Source: CAD feature listing. Evaluate the final solid. Frame: model axes, mm. Face numbers are marked on the shaded views. A direction names the side the tool comes from. Give positions to 0.01 mm unless a question says otherwise; leave off trailing zeros. Write each loop counter-clockwise with the first axis right and the second up, starting at its lowest first coordinate (ties: lowest second). Pieces come first, ordered by that corner, then holes. Notation, with made-up numbers: M 53.25,46.25 L 70.25,46.25 A26 ccw 70.25,85.25 Z; hole C 23,47.5 d4. An arc over 180 degrees is marked long. Return JSON: item names as keys, results as strings.
```python
from build123d import *

# Parameters (mm, degrees)
F2_R     = 12.5
F3_DEPTH = 12.5
F4_R     = 0.5


# Not quite as in the source:
# - the program builds the solid bodies; features that only make, move or delete a surface that nothing else refers to are left out


with BuildPart() as f1:
    # F0 (on Front) → F1 (revolve)
    with BuildSketch(Plane.XZ):
        Polygon((-14, 0), (21, 0), (21, 1.25), (19.85, 2.4), (7.3, 2.4), (6.8, 2.4), (6.4535898385, 3), (4, 3), (4, 4.8), (3.2, 5.6), (-3.2, 5.6), (-4, 4.8), (-4, 3), (-6.4535898385, 3), (-6.8, 2.4), (-7.3, 2.4), (-12.85, 2.4), (-14, 1.25), align=None)
        Polygon((7.3, 2.4), (19.85, 2.4), (19.25, 3), (7.9, 3), align=None)
        Polygon((-12.25, 3), (-12.85, 2.4), (-7.3, 2.4), (-7.9, 3), align=None)
    revolve(axis=Axis((0, 0, 0), (1, 0, 0)))

    # F2 (on Right) → F3 (cut, symmetric)
    with BuildSketch(Plane.YZ):
        Circle(F2_R)
        Polygon((5, -2.8867513459), (0, -5.7735026919), (-5, -2.8867513459), (-5, 2.8867513459), (0, 5.7735026919), (5, 2.8867513459), align=None, mode=Mode.SUBTRACT)
    extrude(amount=F3_DEPTH, both=True, mode=Mode.SUBTRACT)

    # F4
    f4_edges = [f1.edges().sort_by_distance(p)[0] for p in [
        (-4, 0, -3),
        (4, 0, -3),
    ]]
    fillet(f4_edges, radius=F4_R)


solid = f1.part
```
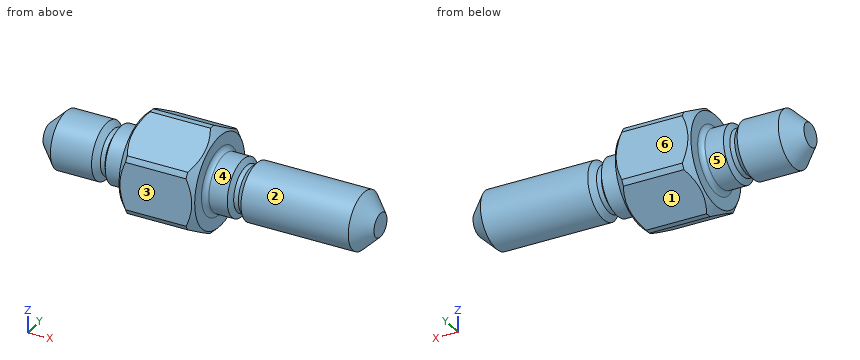
1) Cut plane A-A, the plane x = 0.5. Return the cut outline in (y, z).
Numbers:
{"outline": "M -5,-2.52 A5.6 ccw -4.68,-3.07 L -0.32,-5.59 A5.6 ccw 0.32,-5.59 L 4.68,-3.07 A5.6 ccw 5,-2.52 L 5,2.52 A5.6 ccw 4.68,3.07 L 0.32,5.59 A5.6 ccw -0.32,5.59 L -4.68,3.07 A5.6 ccw -5,2.52 Z"}
2) Set-up query: the marked faces 4, 5 and 6. Return all of +Z, -Z, +X, -X, +Y, -Y with unobstructed straight access to the full face (end or side cutting, diameter ignored); none if empty.
Numbers:
{"face 4": "+X", "face 5": "-X", "face 6": "+Z, -Z, +X, -X, +Y"}
3) Contact query for flat-ended pins moving along their axis: pin 1 Ø1.5 at (x, y) = (-4, 3.5) entering from +Z; pin 2 Ø1 at (x, z) = (-6, 1.5) entering from +Y; pin 3 Ø3 at (x, y) = (4, -2) entering from +Z. Output: stop coordinate, or through.
Numbers:
{"pin 1": "stops at z = 4.17", "pin 2": "stops at y = 2.83", "pin 3": "stops at z = 5.4"}
4) Cut plane B-B, the plane x = 13. Return the cut outline in (y, z).
Numbers:
{"outline": "C 0,0 d6"}
5) Draft query along Y for the marked faces 1, 2 and 3. Return one class per face: released by +Y, released by -Y, zero draft, split by the parting line, or undercut.
Numbers:
{"face 1": "released by +Y", "face 2": "split by the parting line", "face 3": "released by -Y"}
6) Line query: line 1 (X direction, y = 1, z = 4); line 2 (Z direction, x = 15, y = 1.25); line 3 (Z direction, x = 6, y = -2.75). Output: solid intervals per line, ascending. Write a range as [from, to].
Numbers:
{"line 1": "x = [-4, 4]", "line 2": "z = [-2.73, 2.73]", "line 3": "z = [-1.2, 1.2]"}
